from build123d import *

# Parameters (mm, degrees)
SKETCH1_W           = 37
SKETCH1_H           = 40.5
BOSS_EXTRUDE1_DEPTH = 4
SKETCH2_W           = 10
SKETCH2_H           = 4
BOSS_EXTRUDE2_DEPTH = 4
LPATTERN1_COUNT     = 2
LPATTERN1_PITCH     = 20
SKETCH3_W           = 6.75
SKETCH3_H           = 4
SKETCH3_W_2         = 10
BOSS_EXTRUDE3_DEPTH = 6


with BuildPart() as part:
    # Sketch1 → Boss-Extrude1 (new body)
    with BuildSketch(Plane(origin=(0, 0, 0), x_dir=(1, 0, 0), z_dir=(0, 1, 0))):
        with Locations((18.5, -20.25)):
            Rectangle(SKETCH1_W, SKETCH1_H)
    extrude(amount=BOSS_EXTRUDE1_DEPTH)

    # Sketch2 → Boss-Extrude2 (add, through all)
    with BuildSketch(Plane(origin=(0, 0, 0), x_dir=(-1, 0, 0), z_dir=(0, -1, 0))):
        with Locations((-32, 2)):
            Rectangle(SKETCH2_W, SKETCH2_H)
        with Locations((-32, -42.5)):
            Rectangle(SKETCH2_W, SKETCH2_H)
    boss_extrude2 = extrude(amount=-BOSS_EXTRUDE2_DEPTH)

    # LPattern1: Boss-Extrude2 ×2
    with Locations(*[(-i * LPATTERN1_PITCH, 0, 0) for i in range(1, LPATTERN1_COUNT)]):
        add(boss_extrude2)

    # Sketch3 → Boss-Extrude3 (add)
    with BuildSketch(Plane(origin=(37, 0, 0), x_dir=(0, 0, -1), z_dir=(1, 0, 0))):
        with Locations((0.625, 2)):
            Rectangle(SKETCH3_W, SKETCH3_H)
        with Locations((-12.75, 2)):
            Rectangle(SKETCH3_W_2, SKETCH3_H)
        with Locations((-27.75, 2)):
            Rectangle(SKETCH3_W_2, SKETCH3_H)
        with Locations((-41.125, 2)):
            Rectangle(SKETCH3_W, SKETCH3_H)
    extrude(amount=BOSS_EXTRUDE3_DEPTH)


solid = part.part
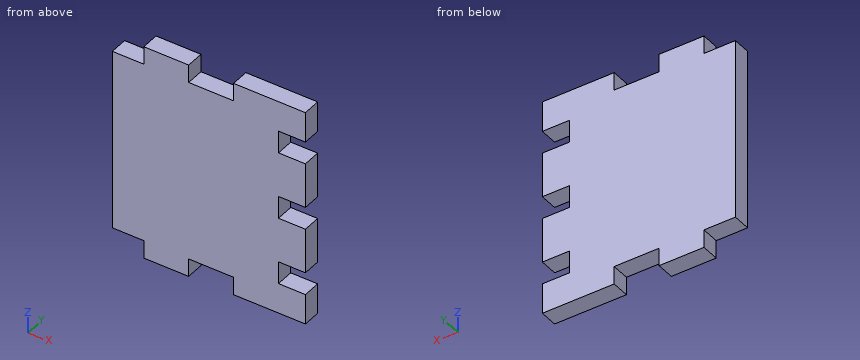
Check sheet for the modelled part. Datum: model origin and axes. Units: mm. Round coordinates to 2 decimals unless told otherwise and drop trailing zeros. Loops run counter-clockwise (first coordinate to the right, second up) from the corner with the lowest first, then second, coordinate; pieces in that order, holes last.
1. Sectioned sample at C-C on z = 34.5. Record the boundary of the cut face in (x, y).
2. Gauge pin test, flat ends, axial feed: pin 1 Ø1.5 at (x, y) = (25, 0.5) entering from -Z; pin 2 Ø1.2 at (y, z) = (2, 20.5) entering from +X; pin 3 Ø2 at (y, z) = (1.5, 42.5) entering from -X. Record the tip position at first contact, or that the pin passes through.
3. Scan lines: probe 1 along Z at (x, y) = (40.5, 2.15); probe 2 along Z at (x, y) = (5.5, 2.25); probe 3 along X at (y, z) = (0.5, 7.5). Record each from-to range of solid material in increasing order.
4. Sectioned sample at A-A on x = 38.5. Record the boundary of the cut face in (y, z).
5. Sectioned sample at B-B on y = 1. Record the boundary of the cut face in (x, z).
6. Sectioned sample at D-D on x = 24.5. Record the boundary of the cut face in (y, z).
Recorded:
1. outline: (0, 0) - (37, 0) - (37, 4) - (0, 4) - close
2. pin 1: stops at z = 0
2. pin 2: stops at x = 37
2. pin 3: stops at x = 7
3. probe 1: z = -4 to 2.75, 7.75 to 17.75, 22.75 to 32.75, 37.75 to 44.5
3. probe 2: z = 0 to 40.5
3. probe 3: x = 0 to 37
4. outline: (0, -4) - (4, -4) - (4, 2.75) - (0, 2.75) - close; (0, 7.75) - (4, 7.75) - (4, 17.75) - (0, 17.75) - close; (0, 22.75) - (4, 22.75) - (4, 32.75) - (0, 32.75) - close; (0, 37.75) - (4, 37.75) - (4, 44.5) - (0, 44.5) - close
5. outline: (0, 0) - (7, 0) - (7, -4) - (17, -4) - (17, 0) - (27, 0) - (27, -4) - (43, -4) - (43, 2.75) - (37, 2.75) - (37, 7.75) - (43, 7.75) - (43, 17.75) - (37, 17.75) - (37, 22.75) - (43, 22.75) - (43, 32.75) - (37, 32.75) - (37, 37.75) - (43, 37.75) - (43, 44.5) - (27, 44.5) - (27, 40.5) - (17, 40.5) - (17, 44.5) - (7, 44.5) - (7, 40.5) - (0, 40.5) - close
6. outline: (0, 0) - (4, 0) - (4, 40.5) - (0, 40.5) - close
